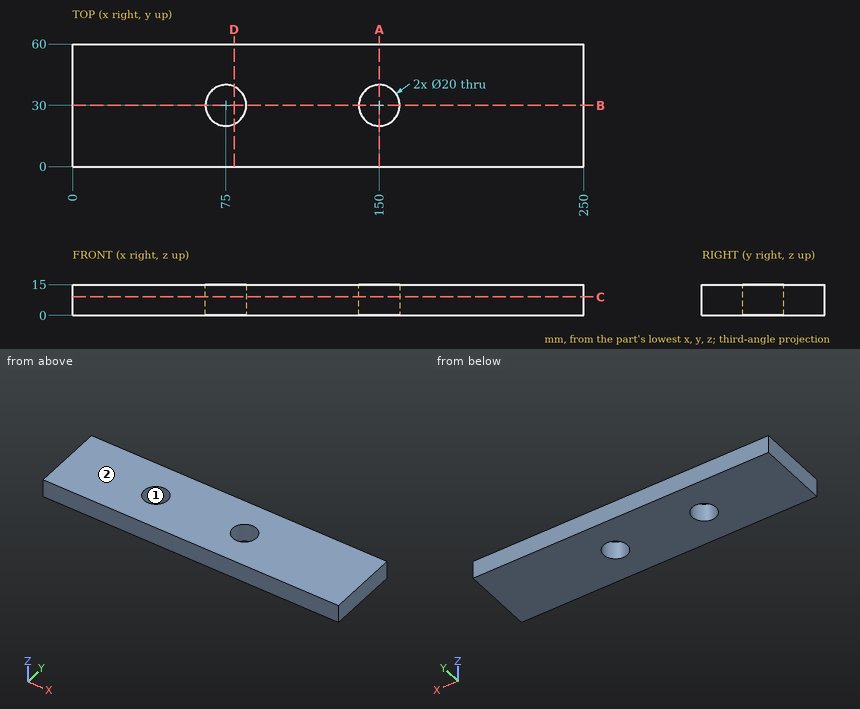
Input: dimensioned drawing with shaded views. Units: mm. Origin: part minimum x, y, z. Round coordinates to 2 decimals unless told otherwise and drop trailing zeros. Order: outer loops, then holes, each group sorted by start corner. A loop starts at its lowest first (then second) coordinate and runs counter-clockwise, first axis right, second up. Notation, with made-up numbers: (-4.75, 76.25) -> (51.25, 76.25) arc R6 cw to (51.25, 86.25) -> close; hole circle Ø6 at (74.25, 57). An arc over 180 degrees is marked (long way). One line per item, written item: value. Start each with the question number.
Q1. Section query A-A (x = 150). Return the cut outline in (y, z), plus the area to 3 significant figures.
Q2. Section query B-B (y = 30). Return the cut outline in (x, z), plus the area to 3 significant figures.
Q3. Material intervals for probe 1 along Y at (x, z) = (150, 4.75); probe 2 along X at (y, z) = (35.5, 13); probe 3 along X at (y, z) = (36, 8.75), sorted ascending.
Q4. Section query D-D (x = 79). Return the cut outline in (y, z).
Q5. Pin query (flat end, axial travel): pin 1 (1.5 mm diameter, centred on x = 96.5, y = 10.5, fed in from -Z); pin 2 (18 mm diameter, centred on x = 150, y = 30, fed in from +Z). Return the tip coordinate at first contact, or that it passes through.
Q6. Draft query along X for the marked faces 1 and 2. Return one class per face: pulls with the +X half, pulls with the -X half, needs draft (parallel to the pull), parting line crosses it, or undercut.
Q7. Section query C-C (z = 9). Return the cut outline in (x, y).
Findings below:
1. outline: (0, 0) -> (20, 0) -> (20, 15) -> (0, 15) -> close; (40, 0) -> (60, 0) -> (60, 15) -> (40, 15) -> close
1. area: 600 mm²
2. outline: (0, 0) -> (65, 0) -> (65, 15) -> (0, 15) -> close; (85, 0) -> (140, 0) -> (140, 15) -> (85, 15) -> close; (160, 0) -> (250, 0) -> (250, 15) -> (160, 15) -> close
2. area: 3,150 mm²
3. probe 1: 0 to 20, 40 to 60
3. probe 2: 0 to 66.65, 83.35 to 141.65, 158.35 to 250
3. probe 3: 0 to 67, 83 to 142, 158 to 250
4. outline: (0, 0) -> (20.83, 0) -> (20.83, 15) -> (0, 15) -> close; (39.17, 0) -> (60, 0) -> (60, 15) -> (39.17, 15) -> close
5. pin 1: z = 0
5. pin 2: through
6. face 1: undercut
6. face 2: needs draft
7. outline: (0, 0) -> (250, 0) -> (250, 60) -> (0, 60) -> close; hole circle Ø20 at (75, 30); hole circle Ø20 at (150, 30)
